Source: CAD feature listing. Evaluate the final solid. Frame: model axes, mm. A direction names the side the tool comes from. Coordinates: 2 decimals unless noted, no trailing zeros. Loops run counter-clockwise (first coordinate to the right, second up) from the corner with the lowest first, then second, coordinate; pieces in that order, holes last. Notation, with made-up numbers: (-5, -34) - (51, -34) arc R27 cw to (51, 0) - close; hole circle Ø2 at (-24.75, -33.75). An arc over 180 degrees is marked (long way). Write item = value, one per line. Start each with the question number.
from build123d import *

# Parameters (mm, degrees)
SKETCH1_R           = 2.5
BOSS_EXTRUDE1_DEPTH = 5
SKETCH3_W           = 55
SKETCH3_H           = 5
BOSS_EXTRUDE2_DEPTH = 129.8
SKETCH4_W           = 55
SKETCH4_H           = 5
BOSS_EXTRUDE3_DEPTH = 67.3
SKETCH5_R           = 2.5
BOSS_EXTRUDE4_DEPTH = 5
CUT_EXTRUDE2_REACH  = 79.3
SKETCH7_W           = 0.569216758
SKETCH7_H           = 67.3
CUT_EXTRUDE3_DEPTH  = 5
CUT_EXTRUDE4_REACH  = 166.8
SKETCH8_W           = 30
SKETCH8_H           = 67.3
BOSS_EXTRUDE5_REACH = 74.3
BOSS_EXTRUDE6_DEPTH = 5
BOSS_EXTRUDE7_DEPTH = 5


with BuildPart() as part:
    # Sketch1 → Boss-Extrude1 (new body)
    with BuildSketch(Plane.XY):
        Polygon((-27.5, 17.5), (-17.5, 27.5), (17.5, 27.5), (27.5, 17.5), (27.5, -27.5), (-27.5, -27.5), align=None)
        Circle(SKETCH1_R, mode=Mode.SUBTRACT)
    extrude(amount=BOSS_EXTRUDE1_DEPTH)

    # Sketch3 → Boss-Extrude2 (add)
    with BuildSketch(Plane.XZ.offset(27.5)):
        with Locations((0, 2.5)):
            Rectangle(SKETCH3_W, SKETCH3_H)
    extrude(amount=BOSS_EXTRUDE2_DEPTH)

    # Sketch4 → Boss-Extrude3 (add)
    with BuildSketch(Plane(origin=(0, 0, 0), x_dir=(-1, 0, 0), z_dir=(0, 0, -1))):
        with Locations((0, -134.8)):
            Rectangle(SKETCH4_W, SKETCH4_H)
    extrude(amount=BOSS_EXTRUDE3_DEPTH)

    # Sketch5 → Boss-Extrude4 (add)
    with BuildSketch(Plane(origin=(0, 0, -67.3), x_dir=(-1, 0, 0), z_dir=(0, 0, -1))):
        Polygon((-27.5, -157.3), (27.5, -157.3), (27.5, 17.5), (17.5, 27.5), (-17.5, 27.5), (-27.5, 17.5), align=None)
        Circle(SKETCH5_R, mode=Mode.SUBTRACT)
    extrude(amount=BOSS_EXTRUDE4_DEPTH)

    # Sketch6 → Cut-Extrude2 (cut, up to next)
    with BuildSketch(Plane.XY.offset(5), mode=Mode.PRIVATE) as cut_extrude2_sk1:
        Polygon((-12.723132969, -157.3), (-27.5, -27.5), (-27.5, -157.3), align=None)
    cut_extrude2_tool1 = extrude(cut_extrude2_sk1.sketch, amount=-CUT_EXTRUDE2_REACH, mode=Mode.PRIVATE) & part.part
    add(cut_extrude2_tool1.solids().sort_by_distance((-22.574378, -114.033333, 5))[0], mode=Mode.SUBTRACT)
    # Sketch6 → Cut-Extrude2 (cut, up to next)
    with BuildSketch(Plane.XY.offset(5), mode=Mode.PRIVATE) as cut_extrude2_sk2:
        Polygon((27.5, -27.5), (12.723132969, -157.3), (27.5, -157.3), align=None)
    cut_extrude2_tool2 = extrude(cut_extrude2_sk2.sketch, amount=-CUT_EXTRUDE2_REACH, mode=Mode.PRIVATE) & part.part
    add(cut_extrude2_tool2.solids().sort_by_distance((22.574378, -114.033333, 5))[0], mode=Mode.SUBTRACT)

    # Sketch7 → Cut-Extrude3 (cut)
    with BuildSketch(Plane.XZ.offset(137.3)):
        with Locations((-15.284608379, -33.65)):
            Rectangle(SKETCH7_W, SKETCH7_H)
        with Locations((15.284608379, -33.65)):
            Rectangle(SKETCH7_W, SKETCH7_H)
    extrude(amount=-CUT_EXTRUDE3_DEPTH, mode=Mode.SUBTRACT)

    # Sketch8 → Cut-Extrude4 (cut, up to next)
    with BuildSketch(Plane.XZ.offset(137.3), mode=Mode.PRIVATE) as cut_extrude4_sk1:
        with Locations((0, -33.65)):
            Rectangle(SKETCH8_W, SKETCH8_H)
    cut_extrude4_tool1 = extrude(cut_extrude4_sk1.sketch, amount=-CUT_EXTRUDE4_REACH, mode=Mode.PRIVATE) & part.part
    add(cut_extrude4_tool1.solids().sort_by_distance((0, -137.3, -33.65))[0], mode=Mode.SUBTRACT)

    # Sketch9 → Boss-Extrude5 (add, up to next)
    with BuildSketch(Plane(origin=(0, 0, 0), x_dir=(-1, 0, 0), z_dir=(0, 0, -1)), mode=Mode.PRIVATE) as boss_extrude5_sk1:
        Polygon((-23.515482696, -62.5), (23.515482696, -62.5), (22.946265938, -67.5), (-22.946265938, -67.5), align=None)
    boss_extrude5_tool1 = extrude(boss_extrude5_sk1.sketch, amount=BOSS_EXTRUDE5_REACH, mode=Mode.PRIVATE) - part.part
    add(boss_extrude5_tool1.solids().sort_by_distance((0, -64.989791, 0))[0])

    # Sketch10 → Boss-Extrude6 (add)
    with BuildSketch(Plane.XY.offset(5)):
        Polygon((27.5, -27.5), (12.723132969, -157.3), (7.78710541, -156.738066079), (22.5, -27.5), align=None)
        Polygon((-27.5, -27.5), (-12.723132969, -157.3), (-7.723132969, -156.730783242), (-22.5, -26.930783242), align=None)
    extrude(amount=BOSS_EXTRUDE6_DEPTH)

    # Sketch11 → Boss-Extrude7 (add)
    with BuildSketch(Plane(origin=(0, 0, -72.3), x_dir=(-1, 0, 0), z_dir=(0, 0, -1))):
        Polygon((-27.5, -27.5), (-12.723132969, -157.3), (-7.78710541, -156.738066079), (-22.5, -27.5), align=None)
        Polygon((27.5, -27.5), (12.723132969, -157.3), (7.755222161, -156.734436383), (22.532089192, -26.934436383), align=None)
    extrude(amount=BOSS_EXTRUDE7_DEPTH)


solid = part.part
Item 1: Material intervals for L1, parallel to Y at x = 0, z = -69.95; L2, parallel to Z at x = -23.5, y = -59; L3, parallel to Z at x = 3.5, y = -17, sorted ascending. Write a range as [from, to].
Item 2: Cut plane B-B (x = 0). Return the cut outline in (y, z), then the cut area to 3 significant figures.
Item 3: Reachability of faces 4 (the flat face through (0, -43, 5)), 5 (the flat face through (10.29, -157.023, 7.465)), 6 (the flat face through (10.29, -157.023, -74.765)), 7 (the flat face through (-24.96, -27.21, 7.46)) from +Z, -Z, +X, -X, +Y, -Y: full face, straight path, thin tool, end or side. Return the list, or none.
Item 4: First-contact query: pin 1 (2.5 mm diameter, centred on x = 24, z = 7, fed in from +Y); pin 2 (16.5 mm diameter, centred on x = -7, y = -25.5, fed in from -Z); pin 3 (3 mm diameter, centred on x = 0.5, z = -62.5, fed in from -Y); pin 4 (4 mm diameter, centred on x = 0, y = 0, fed in from +Z). Flat tips, straight axial feed; report the tip coordinate or a pass-through.
Item 5: Draft query along X for faces 1 (the flat face through (-15.04, -92.74, -74.76)), 2 (the flat face through (-23, 22, -70)), 3 (the flat face through (22, 23, -70)). Return one class per face: released by +X, released by -X, zero draft, split by the parting line, or undercut.
Item 6: Cut plane A-A (y = 0). Return the cut outline in (x, z).
Item 7: Cut plane C-C (y = -29.5). Return the cut outline in (x, z), then the cut area to 3 significant figures.
Item 8: Cut plane D-D (z = -65). Return the cut outline in (x, y).
Responses:
q1.L1 = [-157.3, -2.5], [2.5, 27.5]
q1.L2 = [-77.3, -67.3], [0, 10]
q1.L3 = [-72.3, -67.3], [0, 5]
q2.outline = (-157.3, -72.3) - (-2.5, -72.3) - (-2.5, -67.3) - (-62.5, -67.3) - (-62.5, 0) - (-2.5, 0) - (-2.5, 5) - (-157.3, 5) - (-157.3, 0) - (-67.5, 0) - (-67.5, -67.3) - (-157.3, -67.3) - close; (2.5, -72.3) - (27.5, -72.3) - (27.5, -67.3) - (2.5, -67.3) - close; (2.5, 0) - (27.5, 0) - (27.5, 5) - (2.5, 5) - close
q2.area = 2,130 mm2
q3.face_4 = +Z, +Y
q3.face_5 = +Z, -Y
q3.face_6 = -Z, -Y
q3.face_7 = +Z, -X, +Y
q4.pin_1 = -27.5
q4.pin_2 = -72.3
q4.pin_3 = -67.5
q4.pin_4 = through
q5.face_1 = undercut
q5.face_2 = released by -X
q5.face_3 = released by +X
q6.outline = (-27.5, -72.3) - (-2.5, -72.3) - (-2.5, -67.3) - (-27.5, -67.3) - close; (-27.5, 0) - (-2.5, 0) - (-2.5, 5) - (-27.5, 5) - close; (2.5, -72.3) - (27.5, -72.3) - (27.5, -67.3) - (2.5, -67.3) - close; (2.5, 0) - (27.5, 0) - (27.5, 5) - (2.5, 5) - close
q7.outline = (-27.27, -77.3) - (-22.24, -77.3) - (-22.24, -72.3) - (22.27, -72.3) - (22.27, -77.3) - (27.27, -77.3) - (27.27, -67.3) - (-27.27, -67.3) - close; (-27.27, 0) - (27.27, 0) - (27.27, 10) - (22.27, 10) - (22.27, 5) - (-22.21, 5) - (-22.21, 10) - (-27.27, 10) - close
q7.area = 646 mm2
q8.outline = (-23.52, -62.5) - (-22.95, -67.5) - (22.95, -67.5) - (23.52, -62.5) - close
